Verification items for this drawing (mm, ordinates from the low corner). A direction names the side the tool comes from. Round coordinates to 2 decimals unless told otherwise and drop trailing zeros. Write each loop counter-clockwise with the first axis right and the second up, starting at its lowest first coordinate (ties: lowest second). Pieces come first, ordered by that corner, then holes.
Item 1: Cross-section at D-D (x = 4.45). Enter the section's corners in (y, z).
Item 2: Scan lines: probe 1 along X at (y, z) = (3.8, 4.25); probe 2 along Z at (x, y) = (0.95, 2.95). Record each from-to range of solid material in increasing order.
Item 3: Access from +Z, -Z, +X, -X, +Y, -Y to the whole of each face (thin tool, end or side, straight path). Record for the marked faces 1, 2, 3 and 4.
Item 4: Cross-section at B-B (y = 2.5). Enter the section's corners in (x, z).
Item 5: Depth check by flat-ended pin: P1, Ø0.9, axis at x = 2, z = 21.5, coming from the +Y side; P2, Ø2.5, axis at x = 3, z = 23, coming from the -Y side; P3, Ø2.5, axis at x = 1.5, y = 2, coming from the -Z side; P4, Ø3, axis at y = 3, z = 3, coming from the +X side. Enter the tip coordinate at first touch or a pass-through.
Item 6: Cross-section at A-A (x = 2.5). Enter the section's corners in (y, z), then the cut area to 3 significant figures.
Item 7: Cross-section at C-C (z = 7.75). Enter the section's corners in (x, y), then the cut area to 3 significant figures.
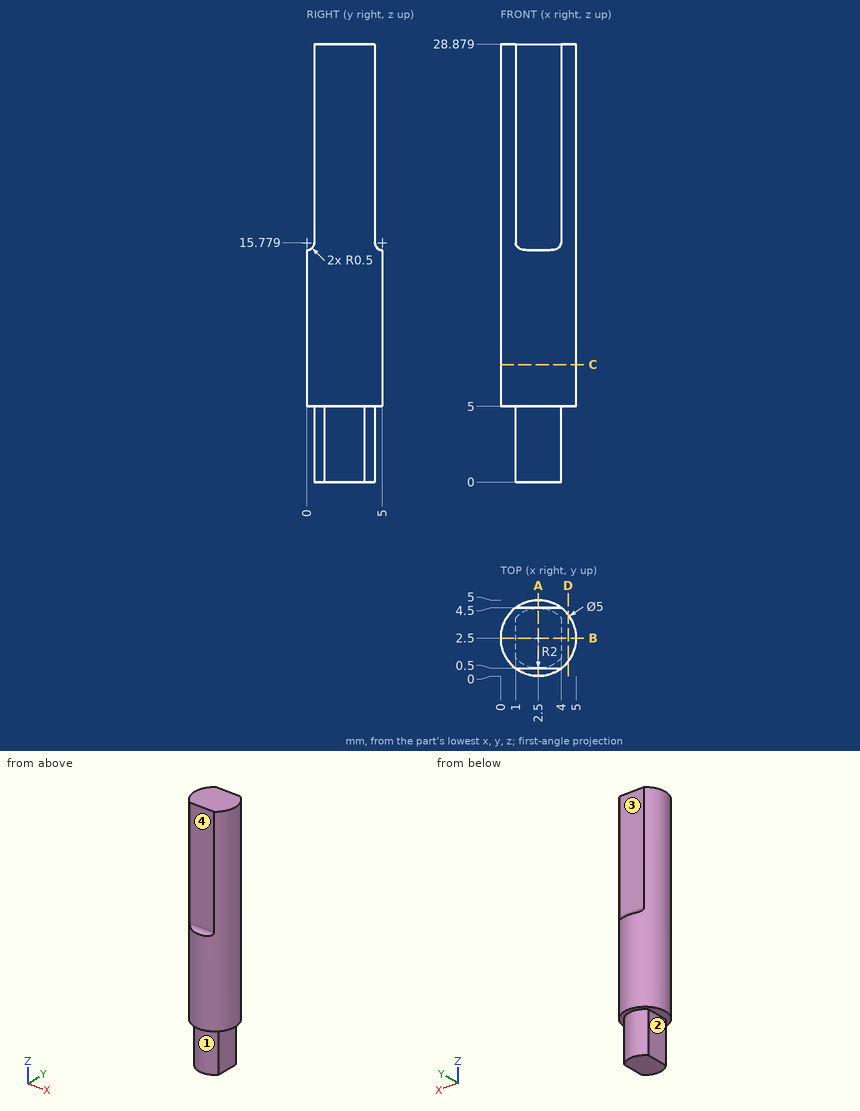
Resolved:
1. outline: (0.94, 5) - (4.06, 5) - (4.06, 28.88) - (0.94, 28.88) - close
2. probe 1: x = 1 to 4
2. probe 2: z = 5 to 28.88
3. face 1: -Z, -Y
3. face 2: -Z, -X, +Y, -Y
3. face 3: +Z, +X, -X, +Y
3. face 4: +Z, +X, -X, -Y
4. outline: (0, 5) - (1, 5) - (1, 0) - (4, 0) - (4, 5) - (5, 5) - (5, 28.88) - (0, 28.88) - close
5. P1: stops at y = 4.5
5. P2: stops at y = 0.5
5. P3: stops at z = 0
5. P4: stops at x = 4
6. outline: (0, 5) - (0.5, 5) - (0.5, 0) - (4.5, 0) - (4.5, 5) - (5, 5) - (5, 15.28) arc R0.5 cw to (4.5, 15.78) - (4.5, 28.88) - (0.5, 28.88) - (0.5, 15.78) arc R0.5 cw to (0, 15.28) - close
6. area: 126 mm2
7. outline: circle Ø5 at (2.5, 2.5)
7. area: 19.6 mm2
